Input: part model. Units: mm. Frame: model coordinates. Face numbers are marked on the shaded views. A direction names the side the tool comes from. Round coordinates to 2 decimals unless told otherwise and drop trailing zeros. Loops run counter-clockwise (first coordinate to the right, second up) from the corner with the lowest first, then second, coordinate; pieces in that order, holes last. Notation, with made-up numbers: (26.25, 13.25) - (66.25, 13.25) arc R25 cw to (66.25, 45.25) - close; hole circle Ø4 at (-39.75, -35.75). An arc over 180 degrees is marked (long way). One line per question, with ' | ' between items. Start each with the question number.
from build123d import *

# Parameters (mm, degrees)
SKETCH1_R           = 25
SKETCH1_R_2         = 3
BOSS_EXTRUDE1_DEPTH = 3
SKETCH2_R           = 7.5
BOSS_EXTRUDE2_DEPTH = 10
BOSS_EXTRUDE3_DEPTH = 35
SKETCH4_R           = 1.25
CUT_EXTRUDE1_DEPTH  = 10
SKETCH5_R           = 12.5
SKETCH5_R_2         = 11
BOSS_EXTRUDE4_DEPTH = 0.5
SKETCH6_R           = 4.5
CUT_EXTRUDE2_DEPTH  = 1.5


with BuildPart() as part:
    # Sketch1 → Boss-Extrude1 (new body)
    with BuildSketch(Plane.XY):
        Circle(SKETCH1_R)
        with Locations((0, 18.75)):
            Circle(SKETCH1_R_2, mode=Mode.SUBTRACT)
        with Locations((16.237976321, -9.375)):
            Circle(SKETCH1_R_2, mode=Mode.SUBTRACT)
        with Locations((-16.237976321, -9.375)):
            Circle(SKETCH1_R_2, mode=Mode.SUBTRACT)
    extrude(amount=BOSS_EXTRUDE1_DEPTH)

    # Sketch2 → Boss-Extrude2 (add)
    with BuildSketch(Plane(origin=(0, 0, 0), x_dir=(-1, 0, 0), z_dir=(0, 0, -1))):
        with Locations(Location((0, 0, 0), (0, 0, 180))):
            Circle(SKETCH2_R)
    extrude(amount=BOSS_EXTRUDE2_DEPTH)

    # Sketch3 → Boss-Extrude3 (add)
    with BuildSketch(Plane(origin=(0, 0, -10), x_dir=(-1, 0, 0), z_dir=(0, 0, -1))):
        Polygon((0, -6.92820323), (6, -3.464101615), (6, 3.464101615), (0, 6.92820323), (-6, 3.464101615), (-6, -3.464101615), align=None)
    extrude(amount=BOSS_EXTRUDE3_DEPTH)

    # Sketch4 → Cut-Extrude1 (cut)
    with BuildSketch(Plane(origin=(0, 0, -45), x_dir=(-1, 0, 0), z_dir=(0, 0, -1))):
        Circle(SKETCH4_R)
    extrude(amount=-CUT_EXTRUDE1_DEPTH, mode=Mode.SUBTRACT)

    # Sketch5 → Boss-Extrude4 (add)
    with BuildSketch(Plane(origin=(0, 0, 0), x_dir=(-1, 0, 0), z_dir=(0, 0, -1))):
        with Locations(Location((0, 0, 0), (0, 0, 180))):
            Circle(SKETCH5_R)
        Circle(SKETCH5_R_2, mode=Mode.SUBTRACT)
    extrude(amount=BOSS_EXTRUDE4_DEPTH)

    # Sketch6 → Cut-Extrude2 (cut)
    with BuildSketch(Plane(origin=(0, 0, 0), x_dir=(-1, 0, 0), z_dir=(0, 0, -1))):
        with Locations((0, 18.75)):
            Circle(SKETCH6_R)
        with Locations((16.237976321, -9.375)):
            Circle(SKETCH6_R)
        with Locations((-16.237976321, -9.375)):
            Circle(SKETCH6_R)
    extrude(amount=-CUT_EXTRUDE2_DEPTH, mode=Mode.SUBTRACT)


solid = part.part
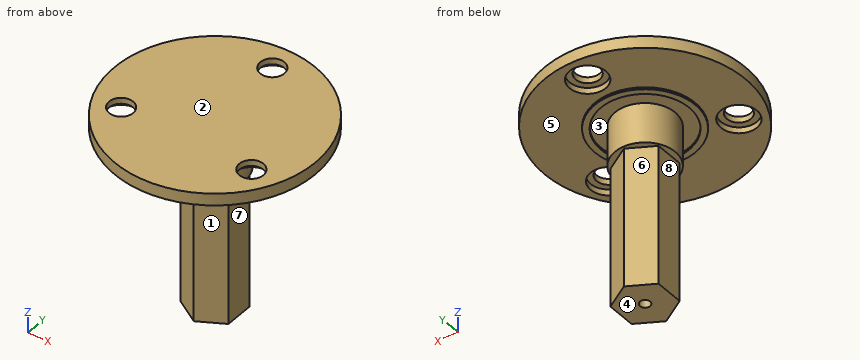
(1) Section B-B, the plane y = -8.5. Output: boundary loops of the cut face in (x, z), plus the area to 3 significant figures.
(2) Section C-C, the plane y = 18.75. Output: boundary loops of the cut face in (x, z), plus the area to 3 significant figures.
(3) Line query: line 1 along Y through (x, z) = (0, -0.3); line 2 along Y through (x, z) = (0, 2); line 3 along X through (y, z) = (-2, -17). Output: solid intervals per line, ascending. Write a range as from..to.
(4) Section D-D, the plane z = -27. Output: boundary loops of the cut face in (x, y), plus the area to 3 significant figures.
(5) Section A-A, the plane z = -41. Output: boundary loops of the cut face in (x, y).
(6) Reachability of the marked faces 4, 5, 6, 7 and 8 from +Z, -Z, +X, -X, +Y, -Y: full face, straight path, thin tool, end or side. Return the list, or none.
(7) Pin query (flat end, axial travel): P1, Ø9.5, axis at x = 16.24, y = -9.38, coming from the -Z side; P2, Ø2, axis at y = -2, z = -26, coming from the +X side; P3, Ø5.5, axis at x = 0, y = 18.75, coming from the -Z side; P4, Ø12, axis at y = 6, z = -8.5, coming from the +X side. Return the tip coordinate at first contact, or that it passes through.
(8) Pull-direction query (X, two-part tool) for the marked faces 1, 2 and 3; classes: released by +X, released by -X, zero draft, split by the parting line, or undercut.
Derived:
1) outline: (-23.51, 0) - (-20.65, 0) - (-20.65, 1.5) - (-19.11, 1.5) - (-19.11, 3) - (-23.51, 3) - close; (-13.37, 1.5) - (-11.82, 1.5) - (-11.82, 0) - (-9.17, 0) - (-9.17, -0.5) - (-6.98, -0.5) - (-6.98, 0) - (6.98, 0) - (6.98, -0.5) - (9.17, -0.5) - (9.17, 0) - (11.82, 0) - (11.82, 1.5) - (13.37, 1.5) - (13.37, 3) - (-13.37, 3) - close; (19.11, 1.5) - (20.65, 1.5) - (20.65, 0) - (23.51, 0) - (23.51, 3) - (19.11, 3) - close | area: 99.5 mm²
2) outline: (-16.54, 0) - (-4.5, 0) - (-4.5, 1.5) - (-3, 1.5) - (-3, 3) - (-16.54, 3) - close; (3, 1.5) - (4.5, 1.5) - (4.5, 0) - (16.54, 0) - (16.54, 3) - (3, 3) - close | area: 76.7 mm²
3) line 1: y = -12.5..-11, -7.5..7.5, 11..12.5 | line 2: y = -25..15.75, 21.75..25 | line 3: x = -6..6
4) outline: (-6, -3.46) - (0, -6.93) - (6, -3.46) - (6, 3.46) - (0, 6.93) - (-6, 3.46) - close | area: 125 mm²
5) outline: (-6, -3.46) - (0, -6.93) - (6, -3.46) - (6, 3.46) - (0, 6.93) - (-6, 3.46) - close; hole circle Ø2.5 at (0, 0)
6) face 4: -Z, +X, -X, +Y, -Y | face 5: -Z | face 6: -Z, -X, +Y | face 7: -Z, +X, +Y, -Y | face 8: -Z, -X, +Y, -Y
7) P1: stops at z = 0 | P2: stops at x = 6 | P3: passes through | P4: stops at x = 7.5
8) face 1: released by +X | face 2: zero draft | face 3: undercut
